The model under review builds one solid part; all positions refer to its coordinate system, in mm. Round coordinates to 2 decimals unless told otherwise and drop trailing zeros. Order: outer loops, then holes, each group sorted by start corner. A loop starts at its lowest first (then second) coordinate and runs counter-clockwise, first axis right, second up. Notation, with made-up numbers: (-39, 50) -> (-26, 50) arc R22 ccw to (-26, 57) -> close; hole circle Ø10 at (67.25, 45). An arc over 180 degrees is marked (long way). Put each result on its own line as item: value. Start each with the question number.
from build123d import *

# Parameters (mm, degrees)
SKETCH1_W                 = 38.1
SKETCH1_H                 = 34.925
BOSS_EXTRUDE1_DEPTH       = 2.38125
SKETCH5_W                 = 101.6
SKETCH5_H                 = 90.17
BOSS_EXTRUDE2_DEPTH       = 2.38125
CUT_EXTRUDE2_REACH        = 121.042
SKETCH6_R                 = 4.7625
F_8_CLEARANCE_HOLE1_D     = 4.3053
F_8_CLEARANCE_HOLE1_DEPTH = 12.7
F_8_CLEARANCE_HOLE1_TIP   = 1.293442612
SKETCH11_W                = 31.75
SKETCH11_H                = 12.7
BOSS_EXTRUDE3_DEPTH       = 2.38125
FILLET3_R                 = 3.175
FILLET4_R                 = 12.7


with BuildPart() as part:
    # Sketch1 → Boss-Extrude1 (new body)
    with BuildSketch(Plane.XY):
        Rectangle(SKETCH1_W, SKETCH1_H)
    extrude(amount=BOSS_EXTRUDE1_DEPTH)

    # Sketch5 → Boss-Extrude2 (add)
    with BuildSketch(Plane.XY.offset(2.38125)):
        with Locations((0, -62.5475)):
            Rectangle(SKETCH5_W, SKETCH5_H)
    extrude(amount=-BOSS_EXTRUDE2_DEPTH)

    # Sketch6 → Cut-Extrude2 (cut, up to next)
    with BuildSketch(Plane(origin=(0, 0, 0), x_dir=(-1, 0, 0), z_dir=(0, 0, -1)), mode=Mode.PRIVATE) as cut_extrude2_sk1:
        with Locations((0, 2.6543)):
            Circle(SKETCH6_R)
    cut_extrude2_tool1 = extrude(cut_extrude2_sk1.sketch, amount=-CUT_EXTRUDE2_REACH, mode=Mode.PRIVATE) & part.part
    add(cut_extrude2_tool1.solids().sort_by_distance((0, 2.6543, 0))[0], mode=Mode.SUBTRACT)

    # #8 Clearance Hole1
    with Locations(Plane(origin=(0, 0, 0), x_dir=(-1, 0, 0), z_dir=(0, 0, -1))):
        with Locations((-8.255, -9.8425), (8.255, -9.8425), (-14.2875, 9.2075), (14.2875, 9.2075)):
            Hole(F_8_CLEARANCE_HOLE1_D / 2, depth=F_8_CLEARANCE_HOLE1_DEPTH)
            with Locations((0, 0, -(F_8_CLEARANCE_HOLE1_DEPTH + F_8_CLEARANCE_HOLE1_TIP / 2))):  # 118° drill point
                Cone(0, F_8_CLEARANCE_HOLE1_D / 2, F_8_CLEARANCE_HOLE1_TIP, mode=Mode.SUBTRACT)

    # Sketch11 → Boss-Extrude3 (add)
    with BuildSketch(Plane.XY.offset(2.38125)):
        with Locations((-34.925, -11.1125)):
            Rectangle(SKETCH11_W, SKETCH11_H)
        with Locations((34.925, -11.1125)):
            Rectangle(SKETCH11_W, SKETCH11_H)
    extrude(amount=-BOSS_EXTRUDE3_DEPTH)

    # Fillet3
    fillet3_edges = [part.edges().sort_by_distance(p)[0] for p in [
        (-50.8, -107.6325, 1.190625),
        (50.8, -107.6325, 1.190625),
        (-19.05, 17.4625, 1.190625),
        (19.05, 17.4625, 1.190625),
        (50.8, -4.7625, 1.190625),
        (-50.8, -4.7625, 1.190625),
    ]]
    fillet(fillet3_edges, radius=FILLET3_R)

    # Fillet4
    fillet4_edges = [part.edges().sort_by_distance(p)[0] for p in [
        (19.05, -4.7625, 1.190625),
        (-19.05, -4.7625, 1.190625),
    ]]
    fillet(fillet4_edges, radius=FILLET4_R)


solid = part.part
Q1. Clearance check with flat-ended pins moving along their axes: pin 1 Ø1.2 at (x, z) = (-42, 0.5) entering from +Y; pin 2 Ø4 at (x, y) = (8.26, -9.84) entering from -Z; pin 3 Ø0.7 at (y, z) = (11, 1.5) entering from -X; pin 4 Ø1.2 at (y, z) = (12.5, 1) entering from +X. State where each tip first meets the part, or that it passes through.
Q2. Take a section at A-A on x = 0. Give the boundary of the cut face in (y, z).
Q3. Draft analysis for pull direction X (two halves, no side actions). For faces 1 (the face through (16.34, 9.85, 1.21)), 2 (the face through (-49.895, -5.717, 1.174)), 3 (the face through (49.89, -106.68, 1.17)), state which applies: +X half, -X half, draft (parallel to the pull), parting line (faces both ways), or undercut.
Q4. Wall thickness on probe 1 along Y at (x, z) = (0, 0.45); probe 2 along Y at (x, z) = (35, 2.1); probe 3 along Y at (x, z) = (2, 0.2): over which ranges is each line inside the solid? List them lowest first. Write a range as [from, to].
Q5. Take a section at C-C on x = 38. Give the boundary of the cut face in (y, z), and give its area (3 significant figures).
Q6. Take a section at B-B on z = 0.65. State how many separate pieces and enclosed holes the cut face has, and give its area (3 significant figures).
Calculated:
1. pin 1: stops at y = -4.76
1. pin 2: passes through
1. pin 3: stops at x = -19.05
1. pin 4: stops at x = 19.05
2. outline: (-107.63, 0) -> (-2.11, 0) -> (-2.11, 2.38) -> (-107.63, 2.38) -> close; (7.42, 0) -> (17.46, 0) -> (17.46, 2.38) -> (7.42, 2.38) -> close
3. face 1: undercut
3. face 2: -X half
3. face 3: +X half
4. probe 1: y = [-107.63, -2.11], [7.42, 17.46]
4. probe 2: y = [-107.63, -4.76]
4. probe 3: y = [-107.63, -1.67], [6.98, 17.46]
5. outline: (-107.63, 0) -> (-4.76, 0) -> (-4.76, 2.38) -> (-107.63, 2.38) -> close
5. area: 245 mm²
6. separate pieces: 1
6. enclosed holes: 5
6. area: 11,200 mm²
